Read the model definition and answer for the solid it produces. Units are mm, in the model's axes. A direction names the side the tool comes from. Coordinates: 2 decimals unless noted, no trailing zeros. Answer as a JSON object with one key per item and string values. Group by question number.
1) Given pin 1 (12 mm diameter, centred on y = 20, z = 18.5, fed in from -X); pin 2 (13 mm diameter, centred on x = -31.75, z = -31.75, fed in from +Y); pin 3 (24.5 mm diameter, centred on x = 7, z = -11, fed in from +Y), each flat-ended and moving along its own axis, determine where each tip first touches the part or whether it passes through.
2) A tool of negligible diameter and unlimited length cuts with its end or side. For faces 5 (the flat face through (-21.68, 9.17, -10.11)), 6 (the flat face through (-16.1, 22.2, -16.1)), 7 (the cylindrical face through (-0.1, 8.1, 38.2)), from which of +Z, -Z, +X, -X, +Y, -Y can it reach the whole face along a straight path? Write none if from no direction.
3) Determine the mould class of faces 1 (the flat face through (0, 17, 33.5)), 2 (the flat face through (42.85, 5, 1)), 3 (the flat face through (1, 5, -42.85)), 4 (the flat face through (23.4, 20.25, 0.3)) for opening direction Z: released by +Z, released by -Z, zero draft, split by the parting line, or undercut.
4) Consider L1, parallel to Z at x = 31.75, y = 6; L2, parallel to Z at x = -29, y = 7.75. Determine where each line is inside the solid, lowest interval first.
5) Section A-A on y = 4.25 is taken. Count the separate pieces of the cut face and the enclosed holes in it, and give its area (3 significant figures).
Autodesk Inventor part; units mm, degrees
ref_plane "brg_XY" through (0, 12.9, 0) normal (0, 1, 0) x (1, 0, 0)
ref_plane "brg_YZ" through (0, 12.9, 0) normal (1, 0, 0) x (0, 0, -1)
ref_plane "brg_ZX" through (0, 12.9, 0) normal (0, 0, -1) x (0, 1, 0)
sketch "Sketch_1" plane through (0, 0, 0) normal (0, 0, 1) x (1, 0, 0)
  line L0 (0, 0) -> (0, 25.8)
  arc A0 (21.3361, 5.55) -> (21.0734, 25.8) centre (0, 15.4) ccw
  line L1 (21.3361, 5.55) -> (24.8875, 5.55)
  line L2 (24.8875, 5.55) -> (24.8875, 0)
  line L3 (24.8875, 0) -> (85.7, 0)
  line L4 (85.7, 0) -> (85.7, 9.1)
  arc A1 (85.7, 9.1) -> (83.7, 11.1) centre (83.7, 9.1) ccw
  line L5 (83.7, 11.1) -> (33.4994, 11.1)
  arc A2 (33.4994, 11.1) -> (30.2815, 25.2277) centre (0, 10.9) ccw
  arc A3 (30.2815, 25.2277) -> (29.3775, 25.8) centre (29.3775, 24.8) ccw
  line L6 (29.3775, 25.8) -> (21.0734, 25.8)
revolve "Revolution1" add sketch "Sketch_1" angle 360 about axis through (0, 0, 0) along (0, -1, 0)
sketch "Sketch_6" plane through (0, 0, 0) normal (0, 1, 0) x (-1, 0, 0)
  circle A0 centre (0, 0) radius 87.7
  arc A1 (42.85, 37.3) -> (37.3, 42.85) centre (37.3, 37.3) ccw
  line L0 (37.3, 42.85) -> (-37.3, 42.85)
  arc A2 (-37.3, 42.85) -> (-42.85, 37.3) centre (-37.3, 37.3) ccw
  line L1 (-42.85, 37.3) -> (-42.85, -37.3)
  arc A3 (-42.85, -37.3) -> (-37.3, -42.85) centre (-37.3, -37.3) ccw
  line L2 (-37.3, -42.85) -> (37.3, -42.85)
  arc A4 (37.3, -42.85) -> (42.85, -37.3) centre (37.3, -37.3) ccw
  line L3 (42.85, -37.3) -> (42.85, 37.3)
extrude "Extrusion1" cut sketch "Sketch_6" along normal blind 25.8
sketch "Sketch_7" plane through (0, 0, 42.85) normal (0, 0, 1) x (1, 0, 0)
  arc A0 (-5.55, 10.2565) -> (5.55, 10.2565) centre (0, 16.32) ccw
  line L0 (5.55, 10.2565) -> (5.55, 11.1)
  line L1 (5.55, 11.1) -> (-5.55, 11.1)
  line L2 (-5.55, 11.1) -> (-5.55, 10.2565)
extrude "Extrusion2" cut sketch "Sketch_7" against normal blind 12.85
sketch "Sketch_4" plane through (0, 0, 0) normal (0, 0, 1) x (1, 0, 0)
  line L0 (0, 5.55) -> (0, 20.25)
  line L1 (0, 20.25) -> (24.8875, 20.25)
  line L2 (24.8875, 20.25) -> (24.8875, 5.55)
  line L3 (24.8875, 5.55) -> (0, 5.55)
  line L4 (0, 5.55) -> (0, 20.25)
revolve "Revolution2" cut sketch "Sketch_4" angle 50 mid plane about axis through (0, 5.55, 0) along (0, 1, 0)
sketch "Sketch_5" plane through (0, 0, 0) normal (0, 0, 1) x (1, 0, 0)
  line L0 (0, 14.7) -> (0, -5.55)
  line L1 (0, -5.55) -> (-24.8875, -5.55)
  line L2 (-24.8875, -5.55) -> (-24.8875, 14.7)
  line L3 (-24.8875, 14.7) -> (0, 14.7)
  line L4 (0, 14.7) -> (0, -5.55)
revolve "Revolution3" cut sketch "Sketch_5" angle 50 mid plane about axis through (0, 14.7, 0) along (0, -1, 0)
sketch "Sketch6" plane through (-37.3, 11.1, -42.85) normal (0, 1, 0) x (1, 0, 0)
  point P0 (5.55, -11.1)
hole "Hole1" at (-31.75, 11.1, -31.75) direction (0, -1, 0) diameter 11.1 depth 11.1
pattern_linear "Rectangular Pattern1" count 2 spacing 63.5 along (1, 0, 0) count 2 spacing 63.5 along (0, 0, 1) of "Hole1"
sketch "Sketch_9" plane through (0, 0, 0) normal (0, 0, 1) x (1, 0, 0)
  line L0 (0, 25.8) -> (0, 22.2)
  line L1 (0, 22.2) -> (-24.25, 22.2)
  arc A0 (-25.2242, 23.4257) -> (-24.25, 22.2) centre (-24.25, 23.2) ccw
  arc A1 (-24.9537, 23.834) -> (-25.2242, 23.4257) centre (-24.5423, 23.2677) ccw
  line L2 (-24.9537, 23.834) -> (-24.45, 24.2)
  line L3 (-24.45, 24.2) -> (-24.4698, 24.361)
  line L4 (-24.4698, 24.361) -> (-25.9088, 25.8)
  line L5 (-25.9088, 25.8) -> (0, 25.8)
  line L6 (0, 25.8) -> (0, 22.2)
revolve "Revolution4" cut sketch "Sketch_9" angle 360 about axis through (0, 25.8, 0) along (0, 1, 0)
sketch "Sketch_10" plane through (0, 0, 33.5) normal (0, 0, 1) x (1, 0, 0)
  line L0 (-5.55, 25.8) -> (-5.55, 6.1)
  line L1 (-5.55, 6.1) -> (5.55, 6.1)
  line L2 (5.55, 6.1) -> (5.55, 25.8)
  line L3 (5.55, 25.8) -> (-5.55, 25.8)
extrude "Extrusion3" add sketch "Sketch_10" against normal blind 5.55
ref_plane "brg_XY" through (0, 12.9, 0) normal (0, 1, 0) x (1, 0, 0)
ref_plane "brg_YZ" through (0, 12.9, 0) normal (1, 0, 0) x (0, 0, -1)
ref_plane "brg_ZX" through (0, 12.9, 0) normal (0, 0, -1) x (0, 1, 0)
ref_plane "housing_XY" through (0, 0, 0) normal (0, 1, 0) x (1, 0, 0)
ref_plane "housing_YZ" through (0, 0, 0) normal (1, 0, 0) x (0, 0, -1)
ref_plane "housing_ZX" through (0, 0, 0) normal (0, 0, -1) x (0, 1, 0)
ref_plane "tocover_XY" through (0, 51.2, 0) normal (0, 1, 0) x (1, 0, 0)
ref_plane "tocover_YZ" through (0, 51.2, 0) normal (1, 0, 0) x (0, 0, -1)
ref_plane "tocover_ZX" through (0, 51.2, 0) normal (0, 0, -1) x (0, 1, 0)
properties part number "F4BSS 504-Y-housing"
Worked answers:
{
 "1": {"pin 1": "stops at x = -30.14", "pin 2": "stops at y = 11.1", "pin 3": "stops at y = 25.18"},
 "2": {"face 5": "-Y", "face 6": "+Y", "face 7": "+Z, +Y"},
 "3": {"face 1": "released by +Z", "face 2": "zero draft", "face 3": "released by -Z", "face 4": "undercut"},
 "4": {"L1": "z = -42.85 to -37.3, -26.2 to 26.2, 37.3 to 42.85", "L2": "z = -42.85 to -36.57, -26.93 to 26.93, 36.57 to 42.85"},
 "5": {"separate pieces": "1", "enclosed holes": "5", "area": "4,990 mm²"}
}
